Design review of the part built by this model. Coordinates are the model's own, in mm. Face numbers are marked on the shaded views. A direction names the side the tool comes from. Coordinates: 2 decimals unless noted, no trailing zeros. Write each loop counter-clockwise with the first axis right and the second up, starting at its lowest first coordinate (ties: lowest second). Pieces come first, ordered by that corner, then holes. Notation, with made-up numbers: (-14, 24) - (11, 24) arc R24 ccw to (11, 40) - close; hole circle Ø5 at (-4.5, -5.75). An arc over 180 degrees is marked (long way). One line per item, written item: value.
from build123d import *

# Parameters (mm, degrees)
SKETCH_1_R               = 25
SKETCH_1_R_2             = 15
EXTRUDE_START            = -25
SKETCH_3_R               = 36
SKETCH_3_R_2             = 25
EXTRUDE_2_DEPTH          = 5
SKETCH_4_W               = 10
SKETCH_4_H               = 4
CUT_EXTRUDE_START        = -20
SKETCH_5_R               = 25
CUT_EXTRUDE_1_DEPTH      = 20
EXTRUDE_START_2          = -6
SKETCH_6_R               = 50
SKETCH_6_R_2             = 15
EXTRUDE_3_DEPTH          = 6
CUT_EXTRUDE_2_REACH      = 140.279
SKETCH_7_R               = 5.1
PATTERN_CIRCULAR_1_COUNT = 6


with BuildPart() as part:
    # По траектории1: sweep along a path in Эскиз2
    with BuildLine(Plane(origin=(0, 0, 0), x_dir=(1, 0, 0), z_dir=(0, 1, 0))) as sweep_1_path:
        Line((0, 0), (0, -62.679491924))
        ThreePointArc((0, -62.679491924), (-4.019237886, -77.679491924), (-15, -88.660254038))
        Line((-15, -88.660254038), (-51.961524227, -110))
    # Эскиз1 → По траектории1 (sweep)
    with BuildSketch(Plane.XY):
        Circle(SKETCH_1_R)
        Circle(SKETCH_1_R_2, mode=Mode.SUBTRACT)
    sweep(path=sweep_1_path.line)

    # Эскиз3 → Бобышка-Вытянуть2 (add)
    with BuildSketch(Plane(origin=(0, 0, 0), x_dir=(-1, 0, 0), z_dir=(0, 0, -1)).offset(EXTRUDE_START)):
        Circle(SKETCH_3_R)
        Circle(SKETCH_3_R_2, mode=Mode.SUBTRACT)
    extrude(amount=EXTRUDE_2_DEPTH)

    # Эскиз4 → Вырез-Повернуть1 (revolve, cut)
    with BuildSketch(Plane(origin=(0, 0, 0), x_dir=(1, 0, 0), z_dir=(0, 1, 0)), mode=Mode.PRIVATE) as cut_revolve_1_sk:
        with Locations((27, -18)):
            Rectangle(SKETCH_4_W, SKETCH_4_H)
    revolve(cut_revolve_1_sk.sketch.rotate(Axis((0, 0, 0), (0, 0, 1)), 180), axis=Axis((0, 0, 0), (0, 0, 1)), mode=Mode.SUBTRACT)

    # Эскиз5 → Вырез-Вытянуть1 (cut)
    with BuildSketch(Plane(origin=(0, 0, 0), x_dir=(-1, 0, 0), z_dir=(0, 0, -1)).offset(CUT_EXTRUDE_START)):
        Circle(SKETCH_5_R)
    extrude(amount=CUT_EXTRUDE_1_DEPTH, mode=Mode.SUBTRACT)

    # Эскиз6 → Бобышка-Вытянуть3 (add)
    with BuildSketch(Plane(origin=(0, 0, 20), x_dir=(-1, 0, 0), z_dir=(0, 0, -1)).offset(EXTRUDE_START_2)):
        Circle(SKETCH_6_R)
        Circle(SKETCH_6_R_2, mode=Mode.SUBTRACT)
    extrude(amount=EXTRUDE_3_DEPTH)

    # Эскиз7 → Вырез-Вытянуть2 (cut, up to next)
    with BuildSketch(Plane(origin=(0, 0, 20), x_dir=(-1, 0, 0), z_dir=(0, 0, -1)), mode=Mode.PRIVATE) as cut_extrude_2_sk1:
        with Locations((-41, 0)):
            Circle(SKETCH_7_R)
    cut_extrude_2_tool1 = extrude(cut_extrude_2_sk1.sketch, amount=-CUT_EXTRUDE_2_REACH, mode=Mode.PRIVATE) & part.part
    cut_extrude_2 = cut_extrude_2_tool1.solids().sort_by_distance((41, 0, 20))[0]
    add(cut_extrude_2, mode=Mode.SUBTRACT)

    # Круговой массив1: Вырез-Вытянуть2 ×6 about axis
    pattern_circular_1_axis = Axis((0, 0, 0), (0, 0, 1))
    for i in range(1, PATTERN_CIRCULAR_1_COUNT):
        add(cut_extrude_2.rotate(pattern_circular_1_axis, i * 360 / PATTERN_CIRCULAR_1_COUNT), mode=Mode.SUBTRACT)


solid = part.part
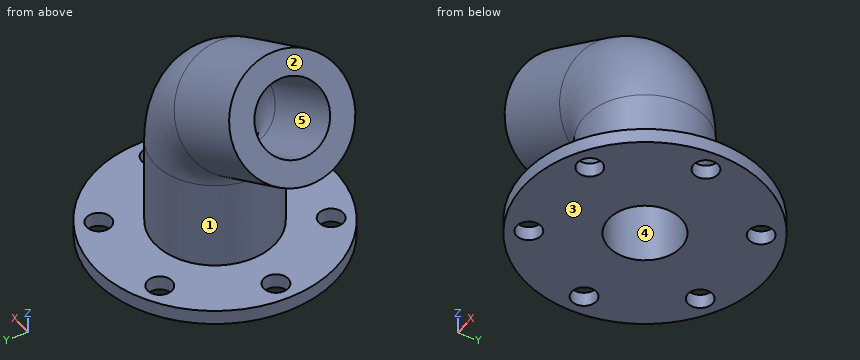
1. Consider section C-C, the plane y = 0. Write out the cut boundary in (x, z).
Answer block:
outline: (-64.46, 88.35) - (-27.5, 67.01) arc R5 cw to (-25, 62.68) - (-25, 26) - (-35.9, 26) - (-35.9, 20) - (-15, 20) - (-15, 62.68) arc R15 ccw to (-22.5, 75.67) - (-59.46, 97.01) - close; (-50, 20) - (-46.1, 20) - (-46.1, 26) - (-50, 26) - close; (-44.46, 122.99) - (-7.5, 101.65) arc R45 cw to (15, 62.68) - (15, 20) - (35.9, 20) - (35.9, 26) - (25, 26) - (25, 62.68) arc R55 ccw to (-2.5, 110.31) - (-39.46, 131.65) - close; (46.1, 20) - (50, 20) - (50, 26) - (46.1, 26) - close
2. For the marked faces 1 and 2, list the 3-axis set-ups (+Z, -Z, +X, -X, +Y, -Y) from which the entire face can be reached by the end or side of a thin tool; tool diameter is ignored.
Answer block:
face 1: none
face 2: +Z, -X, +Y, -Y
3. Wall thickness on line 1 along Y through (x, z) = (0, 43); line 2 along Y through (x, z) = (-20.5, 22.5); line 3 along Y through (x, z) = (-20, 23): over which ranges is each line inside the solid? List them lowest first.
Answer block:
line 1: y = -25 to -15, 15 to 25
line 2: y = -45.6 to -40.61, -30.41 to 30.41, 40.61 to 45.6
line 3: y = -45.83 to -40.58, -30.43 to 30.43, 40.58 to 45.83
4. Insertion check: pin 1 Ø16.5 at (x, y) = (-20.5, 35.51) entering from -Z; pin 2 Ø16.5 at (x, y) = (20.5, 35.51) entering from +Z; pin 3 Ø2 at (x, z) = (-23.5, 91.5) entering from -Y; pin 4 Ø4 at (x, y) = (-20.5, 20.5) entering from +Z. Each pin has a flat end and moves straight along its axis. Give the tip position at first contact, or say it passes through.
Answer block:
pin 1: stops at z = 20
pin 2: stops at z = 26
pin 3: stops at y = -24.99
pin 4: stops at z = 111.5
5. Consider section A-A, the plane x = 41. Write out the cut boundary in (y, z).
Answer block:
outline: (-28.62, 20) - (-5.1, 20) - (-5.1, 26) - (-28.62, 26) - close; (5.1, 20) - (28.62, 20) - (28.62, 26) - (5.1, 26) - close
6. Consider section B-B, the plane z = 45. Write out the cut boundary in (x, y), then the cut area to 3 significant figures.
Answer block:
outline: circle Ø50 at (0, 0); hole circle Ø30 at (0, 0)
area: 1,260 mm^2
7. Mouldability with a two-part tool opening along Z and no side actions: class the marked faces 3, 4 and 5 as released by +Z, released by -Z, zero draft, split by the parting line, or undercut.
Answer block:
face 3: released by -Z
face 4: zero draft
face 5: undercut
8. Consider section D-D, the plane x = -41. Give the number of separate pieces and of enclosed holes in the cut face, then the cut area to 3 significant figures.
Answer block:
separate pieces: 3
enclosed holes: 1
area: 1,680 mm^2
